```python
from build123d import *

# Parameters (mm, degrees)
SKETCH1_R                = 8
BOSS_EXTRUDE1_DEPTH      = 30
SKETCH3_R                = 20
BOSS_EXTRUDE2_DEPTH      = 5
CHAMFER1_SIZE            = 2
SKETCH4_R                = 2.5
CUT_EXTRUDE1_DEPTH       = 71.887234394
CIRPATTERN1_COUNT        = 4
FILLET1_R                = 3
MIRROR1_COPY_1_SKETCH_R  = 2.5
MIRROR1_COPY_1_DEPTH     = 71.887234394
MIRROR1_COPY_2_SKETCH_R  = 2.5
MIRROR1_COPY_2_DEPTH     = 71.887234394
MIRROR1_COPY_3_SKETCH_R  = 2.5
MIRROR1_COPY_3_DEPTH     = 71.887234394
CHAMFER1_OF_MIRROR1_SIZE = 2
FILLET1_OF_MIRROR1_R     = 3


with BuildPart() as part:
    # Sketch1 → Boss-Extrude1 (new, symmetric)
    with BuildSketch(Plane(origin=(0, 0, 0), x_dir=(1, 0, 0), z_dir=(0, 1, 0))):
        with Locations(Location((0, 0, 0), (0, 0, 270))):
            Circle(SKETCH1_R)
    extrude(amount=BOSS_EXTRUDE1_DEPTH, both=True)

    # Sketch3 → Boss-Extrude2 (add)
    with BuildSketch(Plane(origin=(0, 30, 0), x_dir=(1, 0, 0), z_dir=(0, 1, 0))):
        with Locations(Location((0, 0, 0), (0, 0, 270))):
            Circle(SKETCH3_R)
    boss_extrude2 = extrude(amount=BOSS_EXTRUDE2_DEPTH)

    # Chamfer1
    chamfer1_edges = [part.edges().sort_by_distance(p)[0] for p in [
        (0, 35, -20),
    ]]
    chamfer(chamfer1_edges, length=CHAMFER1_SIZE)

    # Sketch4 → Cut-Extrude1 (cut, through all)
    with BuildSketch(Plane(origin=(0, 35, 0), x_dir=(1, 0, 0), z_dir=(0, 1, 0))):
        with Locations(Location((0, 14, 0), (0, 0, 270))):
            Circle(SKETCH4_R)
    cut_extrude1 = extrude(amount=-CUT_EXTRUDE1_DEPTH, mode=Mode.SUBTRACT)

    # CirPattern1: Cut-Extrude1 ×4 about axis
    cirpattern1_axis = Axis((0, 0, 0), (0, 1, 0))
    for i in range(1, CIRPATTERN1_COUNT):
        add(cut_extrude1.rotate(cirpattern1_axis, i * 360 / CIRPATTERN1_COUNT), mode=Mode.SUBTRACT)

    # Fillet1
    fillet1_edges = [part.edges().sort_by_distance(p)[0] for p in [
        (0, 30, -20),
    ]]
    fillet(fillet1_edges, radius=FILLET1_R - 0.0001)  # a hair under: the kernel refuses the full size

    # Mirror1: Boss-Extrude2, Cut-Extrude1 across plane
    add(boss_extrude2.mirror(Plane.ZX))
    add(cut_extrude1.mirror(Plane.ZX), mode=Mode.SUBTRACT)

    # Mirror1 copy 1 sketch → Mirror1 copy 1 (cut, through all)
    with BuildSketch(Plane(origin=(0, -35, 0), x_dir=(0, 0, -1), z_dir=(0, -1, 0))):
        with Locations((0, -14)):
            Circle(MIRROR1_COPY_1_SKETCH_R)
    extrude(amount=-MIRROR1_COPY_1_DEPTH, mode=Mode.SUBTRACT)

    # Mirror1 copy 2 sketch → Mirror1 copy 2 (cut, through all)
    with BuildSketch(Plane(origin=(0, -35, 0), x_dir=(-1, 0, 0), z_dir=(0, -1, 0))):
        with Locations((0, -14)):
            Circle(MIRROR1_COPY_2_SKETCH_R)
    extrude(amount=-MIRROR1_COPY_2_DEPTH, mode=Mode.SUBTRACT)

    # Mirror1 copy 3 sketch → Mirror1 copy 3 (cut, through all)
    with BuildSketch(Plane(origin=(0, -35, 0), x_dir=(0, 0, 1), z_dir=(0, -1, 0))):
        with Locations((0, -14)):
            Circle(MIRROR1_COPY_3_SKETCH_R)
    extrude(amount=-MIRROR1_COPY_3_DEPTH, mode=Mode.SUBTRACT)

    # Chamfer1 of Mirror1
    chamfer1_of_mirror1_edges = [part.edges().sort_by_distance(p)[0] for p in [
        (0, -35, -20),
    ]]
    chamfer(chamfer1_of_mirror1_edges, length=CHAMFER1_OF_MIRROR1_SIZE)

    # Fillet1 of Mirror1
    fillet1_of_mirror1_edges = [part.edges().sort_by_distance(p)[0] for p in [
        (0, -30, -20),
    ]]
    fillet(fillet1_of_mirror1_edges, radius=FILLET1_OF_MIRROR1_R - 0.0001)  # a hair under: the kernel refuses the full size


solid = part.part
```
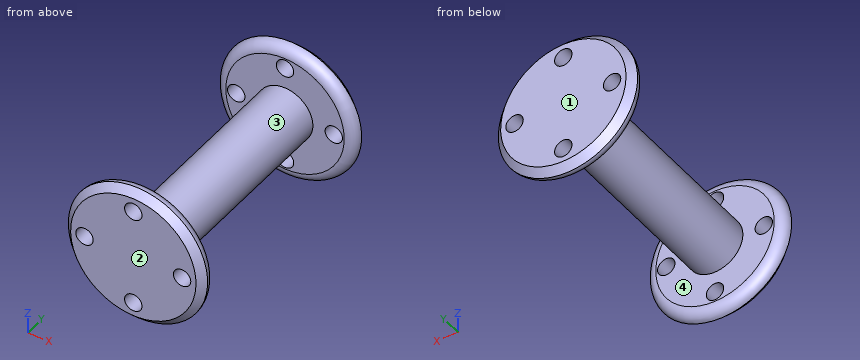
Model file for the job. Use its own axes, mm. Face numbers are marked on the shaded views. Coordinates: 2 decimals unless noted, no trailing zeros. Order: outer loops, then holes, each group sorted by start corner. A loop starts at its lowest first (then second) coordinate and runs counter-clockwise, first axis right, second up. Notation, with made-up numbers: (24, 72.5) -> (61, 72.5) arc R12 cw to (61, 85.5) -> close; hole circle Ø8 at (21.5, 6). An arc over 180 degrees is marked (long way). Answer as a JSON object with one key per item and string values. Group by question number.
1) Cut at B-B, the plane y = 22. Write the cut outline in (x, z), then the cut area to 3 significant figures.
2) Flat gauge pins, fed straight in: pin 1 (4.5 mm diameter, centred on x = -14, z = 0, fed in from -Y); pin 2 (3 mm diameter, centred on x = -0.5, y = 26, fed in from -Z); pin 3 (8 mm diameter, centred on x = -5, y = -19, fed in from -Z); pin 4 (6.5 mm diameter, centred on x = 0, z = 14, fed in from +Y). Where does each tip first touch, or does it go through?
3) Pull direction Y, two halves, no side cores. Call the marked faces 1, 2, 3 and 4: +Y half, -Y half, draft (parallel to the pull), parting line (faces both ways), or undercut.
4) Drill centre lines: L1, parallel to Y at x = 12, z = 6; L2, parallel to Z at x = -14, y = 33.8; L3, parallel to Y at x = -17, z = 6. Where is each one in solid material? Low to high.
5) Cut at A-A, the plane z = 0. Count the separate pieces of the cut face and the enclosed holes in it, then the cut area to 3 significant figures.
Check values:
{
 "1": {"outline": "circle Ø16 at (0, 0)", "area": "201 mm²"},
 "2": {"pin 1": "passes through", "pin 2": "stops at z = -8", "pin 3": "stops at z = -7.94", "pin 4": "stops at y = 35"},
 "3": {"face 1": "+Y half", "face 2": "-Y half", "face 3": "undercut", "face 4": "undercut"},
 "4": {"L1": "y = -35 to -30, 30 to 35", "L2": "z = -13.14 to -2.5, 2.5 to 13.14", "L3": "y = -34.97 to -30.18, 30.18 to 34.97"},
 "5": {"separate pieces": "5", "enclosed holes": "0", "area": "1,240 mm²"}
}
